Here's how the part is built. I have some questions about the finished solid (model axes, mm). Face numbers are marked on the shaded views. A direction names the side the tool comes from. Coordinates: 2 decimals unless noted, no trailing zeros. Loops run counter-clockwise (first coordinate to the right, second up) from the corner with the lowest first, then second, coordinate; pieces in that order, holes last. Notation, with made-up numbers: M 24.5,85.25 L 31.5,85.25 A13 ccw 31.5,91.25 Z; hole C -27.75,1.25 d2. An arc over 180 degrees is marked long. Use CSV: the item, a comma, the result in double quotes. Start each with the question number.
Q1. If we section it at D-D (z = 4): Please give me the cut outline in (x, y), and give its area (3 significant figures).
Q2. For pin 1 Ø4 at (x, z) = (2, 8) entering from +Y; pin 2 Ø2 at (x, z) = (-2, 2) entering from +Y; pin 3 Ø4 at (y, z) = (-1, 9.5) entering from +X, each with a flat end and sliding along its axis, tell me the tip position at first contact or that it passes through.
Q3. If we section it at A-A (y = 0): Please give me the cut outline in (x, z), and give its area (3 significant figures).
Q4. If we mould it in two halves opening along Z, with no side actions, what happens to the marked faces 1, 2 and 3? For each: +Z half, -Z half, draft (parallel to the pull), parting line (faces both ways), or undercut.
Q5. If we section it at C-C (y = -1.75): Please give me the cut outline in (x, z), and give its area (3 significant figures).
Q6. Please list where these lines run through material, in increasing order: probe 1 along Y at (x, z) = (0, 4.75); probe 2 along Z at (x, y) = (-2.25, 3.25); probe 3 along X at (y, z) = (0.75, 7). Write a range as [from, to].
Q7. Which directions (+Z, -Z, +X, -X, +Y, -Y) give clear straight access to the entire face, cutting with the end or side of a thin tool? Please do the marked faces 4 and 5.
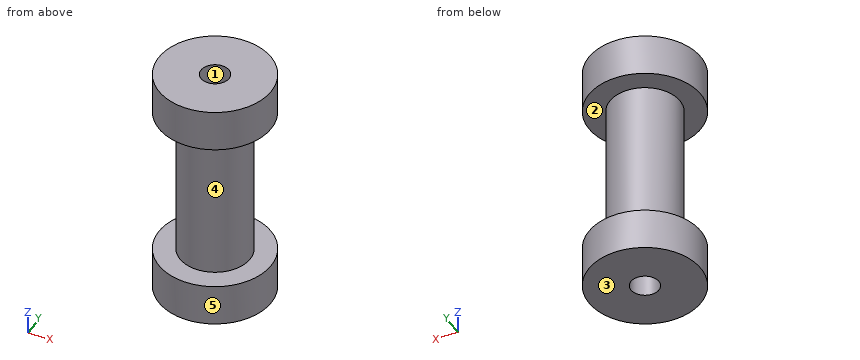
from build123d import *

# Parameters (mm, degrees)
CROQUIS1_R              = 4
SALIENTE_EXTRUIR1_DEPTH = 17
CROQUIS2_R              = 1
CORTAR_EXTRUIR1_DEPTH   = 18.916472867
CROQUIS3_W              = 11
CROQUIS3_H              = 1.5


with BuildPart() as part:
    # Croquis1 → Saliente-Extruir1 (new body)
    with BuildSketch(Plane.XY):
        Circle(CROQUIS1_R)
    extrude(amount=SALIENTE_EXTRUIR1_DEPTH)

    # Croquis2 → Cortar-Extruir1 (cut, through all)
    with BuildSketch(Plane.XY.offset(17)):
        Circle(CROQUIS2_R)
    extrude(amount=-CORTAR_EXTRUIR1_DEPTH, mode=Mode.SUBTRACT)

    # Croquis3 → Cortar-Revolución1 (revolve, cut)
    with BuildSketch(Plane(origin=(0, 0, 0), x_dir=(0, 0, -1), z_dir=(1, 0, 0)), mode=Mode.PRIVATE) as cortar_revoluci_n1_sk:
        with Locations((-8.5, 3.25)):
            Rectangle(CROQUIS3_W, CROQUIS3_H)
    revolve(cortar_revoluci_n1_sk.sketch.rotate(Axis((0, 0, 17), (0, 0, -1)), 90), axis=Axis((0, 0, 17), (0, 0, -1)), mode=Mode.SUBTRACT)


solid = part.part
Results below:
1,outline,"C 0,0 d5; hole C 0,0 d2"
1,area,"16.5 mm^2"
2,pin 1,"y = 2.5"
2,pin 2,"y = 3.87"
2,pin 3,"x = 2.5"
3,outline,"M -4,0 L -1,0 L -1,17 L -4,17 L -4,14 L -2.5,14 L -2.5,3 L -4,3 Z; M 1,0 L 4,0 L 4,3 L 2.5,3 L 2.5,14 L 4,14 L 4,17 L 1,17 Z"
3,area,"69.0 mm^2"
4,face 1,"draft"
4,face 2,"undercut"
4,face 3,"-Z half"
5,outline,"M -3.6,0 L 3.6,0 L 3.6,3 L 1.79,3 L 1.79,14 L 3.6,14 L 3.6,17 L -3.6,17 L -3.6,14 L -1.79,14 L -1.79,3 L -3.6,3 Z"
5,area,"82.4 mm^2"
6,probe 1,"[-2.5, -1], [1, 2.5]"
6,probe 2,"[0, 3], [14, 17]"
6,probe 3,"[-2.38, -0.66], [0.66, 2.38]"
7,face 4,"none"
7,face 5,"+Z, -Z"
